Read the model definition and answer for the solid it produces. Units are mm, in the model's axes. Face numbers are marked on the shaded views. A direction names the side the tool comes from. Coordinates: 2 decimals unless noted, no trailing zeros. Loops run counter-clockwise (first coordinate to the right, second up) from the corner with the lowest first, then second, coordinate; pieces in that order, holes last. Notation, with made-up numbers: (76.5, 64) -> (83.5, 64) arc R8 ccw to (83.5, 70) -> close; hole circle Ø1 at (36, 30). An arc over 180 degrees is marked (long way). Answer in a Markdown table with one row per item.
```python
from build123d import *

# Parameters (mm, degrees)
SKETCH1_R           = 1.5
SKETCH1_W           = 30
SKETCH1_H           = 43
SKETCH1_W_2         = 27.2
SKETCH1_H_2         = 41
SKETCH1_W_3         = 24.5
SKETCH1_H_3         = 21.1
BOSS_EXTRUDE1_DEPTH = 2.1
BOSS_EXTRUDE2_START = 2.1
SKETCH1_3_W         = 27.2
SKETCH1_3_H         = 41
SKETCH1_3_W_2       = 24.5
SKETCH1_3_H_2       = 21.1
BOSS_EXTRUDE2_DEPTH = 2.1
FILLET1_R           = 3
SKETCH1_4_W         = 27.2
SKETCH1_4_H         = 41
SKETCH1_4_W_2       = 24.5
SKETCH1_4_H_2       = 21.1
BOSS_EXTRUDE3_DEPTH = 15
BOSS_EXTRUDE4_START = -15
SKETCH1_5_W         = 24.5
SKETCH1_5_H         = 21.1
BOSS_EXTRUDE4_DEPTH = 2.2


with BuildPart() as part:
    # Sketch1 → Boss-Extrude1 (new body)
    # profile 1 of 4: a face of its own
    with BuildSketch(Plane(origin=(0, 0, 0), x_dir=(0, 0, -1), z_dir=(1, 0, 0))):
        with BuildLine():
            ThreePointArc((-4.5375, 28.390108399), (0, 29.75), (4.5375, 28.390108399))
            Line((4.5375, 28.390108399), (15, 21.5))
            Line((15, 21.5), (-15, 21.5))
            Line((-15, 21.5), (-4.5375, 28.390108399))
        make_face()
        with Locations((0, 25.5)):
            Circle(SKETCH1_R, mode=Mode.SUBTRACT)
    # profile 2 of 4: a face of its own
    with BuildSketch(Plane(origin=(0, 0, 0), x_dir=(0, 0, -1), z_dir=(1, 0, 0))):
        Rectangle(SKETCH1_W, SKETCH1_H)
        Rectangle(SKETCH1_W_2, SKETCH1_H_2, mode=Mode.SUBTRACT)
    # profile 3 of 4: a face of its own
    with BuildSketch(Plane(origin=(0, 0, 0), x_dir=(0, 0, -1), z_dir=(1, 0, 0))):
        Rectangle(SKETCH1_W_2, SKETCH1_H_2)
        Polygon((-12.25, 14.1), (-12.25, 3), (12.25, 3), (12.25, 14.1), (7.35, 19), (-7.35, 19), align=None, mode=Mode.SUBTRACT)
        with Locations((0, -8.45)):
            Rectangle(SKETCH1_W_3, SKETCH1_H_3, mode=Mode.SUBTRACT)
    # profile 4 of 4: a face of its own
    with BuildSketch(Plane(origin=(0, 0, 0), x_dir=(0, 0, -1), z_dir=(1, 0, 0))):
        with BuildLine():
            Line((-15, -21.5), (-4.5375, -28.390108399))
            ThreePointArc((-4.5375, -28.390108399), (0, -29.75), (4.5375, -28.390108399))
            Line((4.5375, -28.390108399), (15, -21.5))
            Line((15, -21.5), (-15, -21.5))
        make_face()
        with Locations((0, -25.5)):
            Circle(SKETCH1_R, mode=Mode.SUBTRACT)
    extrude(amount=BOSS_EXTRUDE1_DEPTH)

    # Sketch1<3> → Boss-Extrude2 (add)
    with BuildSketch(Plane(origin=(0, 0, 0), x_dir=(0, 0, -1), z_dir=(1, 0, 0)).offset(BOSS_EXTRUDE2_START)):
        Rectangle(SKETCH1_3_W, SKETCH1_3_H)
        Polygon((-12.25, 14.1), (-12.25, 3), (12.25, 3), (12.25, 14.1), (7.35, 19), (-7.35, 19), align=None, mode=Mode.SUBTRACT)
        with Locations((0, -8.45)):
            Rectangle(SKETCH1_3_W_2, SKETCH1_3_H_2, mode=Mode.SUBTRACT)
    extrude(amount=BOSS_EXTRUDE2_DEPTH)

    # Fillet1
    fillet1_edges = [part.edges().sort_by_distance(p)[0] for p in [
        (3.15, -20.5, 13.6),
        (3.15, -20.5, -13.6),
        (3.15, 20.5, -13.6),
        (3.15, 20.5, 13.6),
    ]]
    fillet(fillet1_edges, radius=FILLET1_R)

    # Sketch1<4> → Boss-Extrude3 (add)
    with BuildSketch(Plane(origin=(0, 0, 0), x_dir=(0, 0, -1), z_dir=(1, 0, 0))):
        Rectangle(SKETCH1_4_W, SKETCH1_4_H)
        Polygon((-12.25, 14.1), (-12.25, 3), (12.25, 3), (12.25, 14.1), (7.35, 19), (-7.35, 19), align=None, mode=Mode.SUBTRACT)
        with Locations((0, -8.45)):
            Rectangle(SKETCH1_4_W_2, SKETCH1_4_H_2, mode=Mode.SUBTRACT)
    extrude(amount=-BOSS_EXTRUDE3_DEPTH)

    # Sketch1<5> → Boss-Extrude4 (add)
    with BuildSketch(Plane(origin=(0, 0, 0), x_dir=(0, 0, -1), z_dir=(1, 0, 0)).offset(BOSS_EXTRUDE4_START)):
        Polygon((-7.35, 19), (-12.25, 14.1), (-12.25, 3), (12.25, 3), (12.25, 14.1), (7.35, 19), align=None)
        with Locations((0, -8.45)):
            Rectangle(SKETCH1_5_W, SKETCH1_5_H)
    extrude(amount=BOSS_EXTRUDE4_DEPTH)


solid = part.part
```
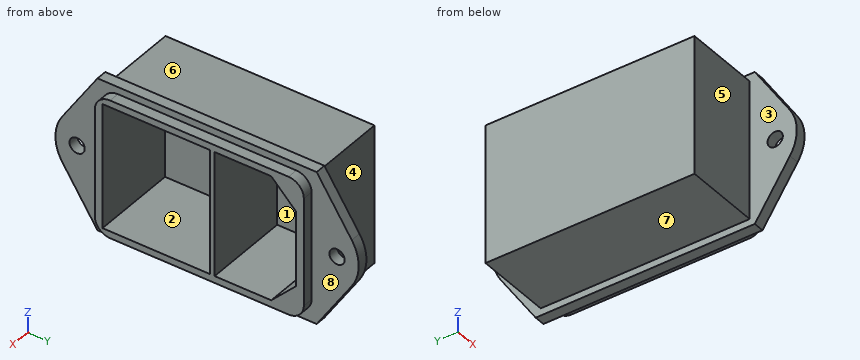
1. A cutting plane is placed at B-B on x = -8.25. Give the vertices of the cut face in (y, z), and give its area (3 significant figures).
A:
| item | result |
|---|---|
| outline | (-20.5, -13.6) -> (20.5, -13.6) -> (20.5, 13.6) -> (-20.5, 13.6) -> close; hole (-19, -12.25) -> (2.1, -12.25) -> (2.1, 12.25) -> (-19, 12.25) -> close; hole (3, -12.25) -> (14.1, -12.25) -> (19, -7.35) -> (19, 7.35) -> (14.1, 12.25) -> (3, 12.25) -> close |
| area | 230 mm2 |
2. A cutting plane is placed at D-D on y = 4.5. Give the vertices of the cut face in (x, z), and give its area (3 significant figures).
A:
| item | result |
|---|---|
| outline | (-15, -13.6) -> (0, -13.6) -> (0, -15) -> (2.1, -15) -> (2.1, -13.6) -> (4.2, -13.6) -> (4.2, -12.25) -> (-12.8, -12.25) -> (-12.8, 12.25) -> (4.2, 12.25) -> (4.2, 13.6) -> (2.1, 13.6) -> (2.1, 15) -> (0, 15) -> (0, 13.6) -> (-15, 13.6) -> close |
| area | 112 mm2 |
3. Given pin 1 Ø0.6 at (x, z) = (3.5, 0.5) entering from -Y; pin 2 Ø4.5 at (x, z) = (0, -2) entering from -Y; pin 3 Ø10 at (x, y) = (-13, -8.5) entering from +Z; pin 4 Ø3.5 at (x, y) = (-2, 6) entering from -Z, each flat-ended and moving along its own axis, determine where each tip first touches the part or whether it passes through.
A:
| item | result |
|---|---|
| pin 1 | stops at y = -20.5 |
| pin 2 | stops at y = -29.75 |
| pin 3 | stops at z = 13.6 |
| pin 4 | stops at z = -13.6 |
4. A cutting plane is placed at A-A on z = 0. Give the vertices of the cut face in (x, y), and give its area (3 significant figures).
A:
| item | result |
|---|---|
| outline | (-15, -20.5) -> (0, -20.5) -> (0, -24) -> (2.1, -24) -> (2.1, -20.5) -> (4.2, -20.5) -> (4.2, -19) -> (-12.8, -19) -> (-12.8, 2.1) -> (4.2, 2.1) -> (4.2, 3) -> (-12.8, 3) -> (-12.8, 19) -> (4.2, 19) -> (4.2, 20.5) -> (2.1, 20.5) -> (2.1, 24) -> (0, 24) -> (0, 20.5) -> (-15, 20.5) -> close; (0, -29.75) -> (2.1, -29.75) -> (2.1, -27) -> (0, -27) -> close; (0, 27) -> (2.1, 27) -> (2.1, 29.75) -> (0, 29.75) -> close |
| area | 183 mm2 |
5. A tool of negligible diameter and unlimited length cuts with its end or side. For the marked faces 5, 6, 7 and 8, from which of +Z, -Z, +X, -X, +Y, -Y can it reach the whole face along a straight path? Write none if from no direction.
A:
| item | result |
|---|---|
| face 5 | +Z, -Z, -X, -Y |
| face 6 | +Z, -X, +Y, -Y |
| face 7 | -Z, -X, +Y, -Y |
| face 8 | +X |
6. The mould has two halves that part along Y. Classify the marked faces 1, 2, 3 and 4: pulls with the +Y half, pulls with the -Y half, needs draft (parallel to the pull), parting line crosses it, or undercut.
A:
| item | result |
|---|---|
| face 1 | undercut |
| face 2 | undercut |
| face 3 | needs draft |
| face 4 | pulls with the +Y half |
7. A cutting plane is placed at C-C on y = 25.5. Give the vertices of the cut face in (x, z), and give its area (3 significant figures).
A:
| item | result |
|---|---|
| outline | (0, -8.93) -> (2.1, -8.93) -> (2.1, -1.5) -> (0, -1.5) -> close; (0, 1.5) -> (2.1, 1.5) -> (2.1, 8.93) -> (0, 8.93) -> close |
| area | 31.2 mm2 |
8. Find the intervals of material crossed by probe 1 along Y at (x, z) = (0.65, 0); probe 2 along Y at (x, z) = (-0.25, -4); probe 3 along Y at (x, z) = (-10, -12.75), in increasing order.
A:
| item | result |
|---|---|
| probe 1 | y = -29.75 to -27, -24 to -19, 2.1 to 3, 19 to 24, 27 to 29.75 |
| probe 2 | y = -20.5 to -19, 2.1 to 3, 19 to 20.5 |
| probe 3 | y = -20.5 to 20.5 |
